The figure shows three views and two pictorial views of one solid part (mm, origin at its lowest corner). Answer the questions. Coordinates: 2 decimals unless noted, no trailing zeros. Write each loop counter-clockwise with the first axis right and the second up, starting at its lowest first coordinate (ties: lowest second). Pieces come first, ordered by that corner, then holes.
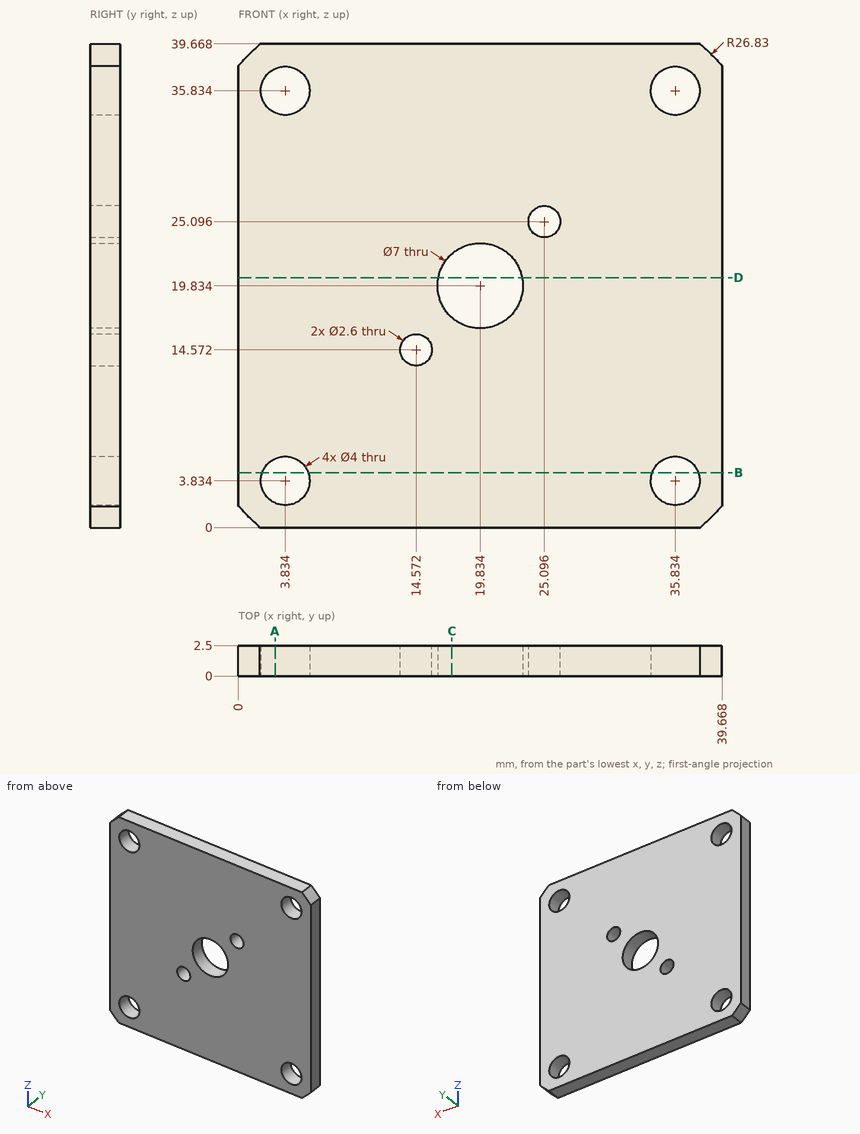
Q1. The part is cut by section C-C, the plane x = 17.5. Write down the section's boundary in (y, z) (1 decimal).
Answers below:
outline: (0, 0) - (2.5, 0) - (2.5, 17.2) - (0, 17.2) - close; (0, 22.4) - (2.5, 22.4) - (2.5, 39.7) - (0, 39.7) - close
Q2. The part is cut by section D-D, the plane z = 20.5. Write down the section's boundary in (x, y).
Answers below:
outline: (0, 0) - (16.4, 0) - (16.4, 2.5) - (0, 2.5) - close; (23.27, 0) - (39.67, 0) - (39.67, 2.5) - (23.27, 2.5) - close
Q3. Find the intervals of material crossed by probe 1 along X at (y, z) = (0.6, 20); probe 2 along X at (y, z) = (1.7, 2) (1 decimal), in increasing order.
Answers below:
probe 1: x = 0 to 16.34, 23.33 to 39.67
probe 2: x = 0 to 3, 4.6 to 35, 36.6 to 39.7
Q4. The part is cut by section B-B, the plane z = 4.5. Write down the section's boundary in (x, y).
Answers below:
outline: (0, 0) - (1.95, 0) - (1.95, 2.5) - (0, 2.5) - close; (5.72, 0) - (33.95, 0) - (33.95, 2.5) - (5.72, 2.5) - close; (37.72, 0) - (39.67, 0) - (39.67, 2.5) - (37.72, 2.5) - close
Q5. The part is cut by section A-A, the plane x = 3. Write down the section's boundary in (y, z).
Answers below:
outline: (0, 0) - (2.5, 0) - (2.5, 2.02) - (0, 2.02) - close; (0, 5.65) - (2.5, 5.65) - (2.5, 34.02) - (0, 34.02) - close; (0, 37.65) - (2.5, 37.65) - (2.5, 39.67) - (0, 39.67) - close
